Source: CAD feature listing. Evaluate the final solid. Frame: model axes, mm. Face numbers are marked on the shaded views. A direction names the side the tool comes from. Give positions to 0.01 mm unless a question says otherwise; leave off trailing zeros. Write each loop counter-clockwise with the first axis right and the second up, starting at its lowest first coordinate (ties: lowest second). Pieces come first, ordered by that corner, then holes. Notation, with made-up numbers: (81.5, -34) -> (94.5, -34) arc R32 cw to (94.5, -7) -> close; hole circle Ø9 at (76.25, 28). An arc over 180 degrees is marked (long way). Use a Markdown table: item, result. Add a question column.
```python
from build123d import *

# Parameters (mm, degrees)
SKETCH_1_W           = 80
SKETCH_1_H           = 150
EXTRUDE_1_DEPTH      = 10
SKETCH_4_R           = 11.25
EXTRUDE_3_DEPTH      = 10
SKETCH_5_R           = 11.25
SKETCH_5_R_2         = 5
EXTRUDE_4_DEPTH      = 4
SKETCH_6_R           = 2.1
CUT_EXTRUDE_1_DEPTH  = 24
SKETCH_7_W           = 3.4
SKETCH_7_H           = 7.5
CUT_EXTRUDE_2_DEPTH  = 24
SKETCH_8_R           = 2.1
CUT_EXTRUDE_3_DEPTH  = 24
SKETCH_9_W           = 80
SKETCH_9_H           = 40
SKETCH_9_R           = 11
SKETCH_9_R_2         = 1.6
EXTRUDE_5_DEPTH      = 10
FILLET_1_R           = 5
SKETCH_10_W          = 3.4
SKETCH_10_H          = 7.5
CUT_EXTRUDE_5_DEPTH  = 10
SKETCH_11_R          = 2.1
CUT_EXTRUDE_6_DEPTH  = 24
SKETCH_12_R          = 2.1
CUT_EXTRUDE_7_DEPTH  = 24
SKETCH_14_W          = 4
SKETCH_14_H          = 2
CUT_EXTRUDE_9_DEPTH  = 10
SKETCH_16_R          = 2.1
CUT_EXTRUDE_10_DEPTH = 11
CUT_EXTRUDE_12_DEPTH = 81
CUT_EXTRUDE_13_DEPTH = 3
SKETCH_20_R          = 1.6
CUT_EXTRUDE_15_DEPTH = 20


with BuildPart() as part:
    # 草圖1 → 填料-伸長1 (new body)
    with BuildSketch(Plane.XY):
        Rectangle(SKETCH_1_W, SKETCH_1_H)
    extrude(amount=EXTRUDE_1_DEPTH)

    # 草圖4 → 填料-伸長3 (add)
    with BuildSketch(Plane.XZ.offset(75)):
        with BuildLine():
            ThreePointArc((-6, 49), (0, 43), (6, 49))
            Line((6, 49), (6, 50))
            Line((6, 50), (29, 50))
            Line((29, 50), (29, 27.881405907))
            ThreePointArc((29, 27.881405907), (30, 21.95), (31, 27.881405907))
            Line((31, 27.881405907), (31, 50))
            Line((31, 50), (40, 50))
            Line((40, 50), (40, 10))
            Line((40, 10), (-40, 10))
            Line((-40, 10), (-40, 50))
            Line((-40, 50), (-31, 50))
            Line((-31, 50), (-31, 27.881405907))
            ThreePointArc((-31, 27.881405907), (-30, 21.95), (-29, 27.881405907))
            Line((-29, 27.881405907), (-29, 50))
            Line((-29, 50), (-6, 50))
            Line((-6, 50), (-6, 49))
        make_face()
        with Locations((0, 25)):
            Circle(SKETCH_4_R, mode=Mode.SUBTRACT)
    extrude(amount=-EXTRUDE_3_DEPTH)

    # 草圖5 → 填料-伸長4 (add)
    with BuildSketch(Plane.XZ.offset(75)):
        with Locations((0, 25)):
            Circle(SKETCH_5_R)
        with Locations((0, 25)):
            Circle(SKETCH_5_R_2, mode=Mode.SUBTRACT)
    extrude(amount=-EXTRUDE_4_DEPTH)

    # 草圖6 → 除料-伸長1 (cut)
    with BuildSketch(Plane(origin=(40, 0, 0), x_dir=(0, 0, -1), z_dir=(1, 0, 0))):
        with Locations((-40, -70)):
            Circle(SKETCH_6_R)
    extrude(amount=-CUT_EXTRUDE_1_DEPTH, mode=Mode.SUBTRACT)

    # 草圖7 → 除料-伸長2 (cut)
    with BuildSketch(Plane.XZ.offset(75)):
        with Locations((-21.943112787, 40)):
            Rectangle(SKETCH_7_W, SKETCH_7_H)
        with Locations((21.943112787, 40)):
            Rectangle(SKETCH_7_W, SKETCH_7_H)
    extrude(amount=-CUT_EXTRUDE_2_DEPTH, mode=Mode.SUBTRACT)

    # 草圖8 → 除料-伸長3 (cut)
    with BuildSketch(Plane.ZY.offset(40)):
        with Locations((40, -70)):
            Circle(SKETCH_8_R)
    extrude(amount=-CUT_EXTRUDE_3_DEPTH, mode=Mode.SUBTRACT)

    # 草圖9 → 填料-伸長5 (add)
    with BuildSketch(Plane(origin=(0, 75, 0), x_dir=(1, 0, 0), z_dir=(0, 1, 0))):
        with Locations((0, -30)):
            Rectangle(SKETCH_9_W, SKETCH_9_H)
        with Locations((0, -25)):
            Circle(SKETCH_9_R, mode=Mode.SUBTRACT)
        with Locations((-21.920310217, -25)):
            Circle(SKETCH_9_R_2, mode=Mode.SUBTRACT)
        with Locations((0, -46.920310217)):
            Circle(SKETCH_9_R_2, mode=Mode.SUBTRACT)
        with Locations((21.920310217, -25)):
            Circle(SKETCH_9_R_2, mode=Mode.SUBTRACT)
    extrude(amount=-EXTRUDE_5_DEPTH)

    # 圓角1
    fillet_1_edges = [part.edges().sort_by_distance(p)[0] for p in [
        (40, 70, 50),
        (-40, 70, 50),
        (40, -70, 50),
        (-40, -70, 50),
    ]]
    fillet(fillet_1_edges, radius=FILLET_1_R)

    # 草圖10 → 除料-伸長5 (cut)
    with BuildSketch(Plane(origin=(0, 75, 0), x_dir=(1, 0, 0), z_dir=(0, 1, 0))):
        with BuildLine():
            Line((-30.992105359, -72.117230176), (-29, -72.117230176))
            Line((-29, -72.117230176), (-29, -27.881405907))
            ThreePointArc((-29, -27.881405907), (-30.004176302, -21.950002859), (-30.992105359, -27.884133658))
            Line((-30.992105359, -27.884133658), (-30.992105359, -72.117230176))
        make_face()
        with BuildLine():
            Line((29.001577897, -72.118320527), (31, -72.118320527))
            Line((31, -72.118320527), (31, -27.881405907))
            ThreePointArc((31, -27.881405907), (29.999164969, -21.950000114), (29.001577897, -27.881953036))
            Line((29.001577897, -27.881953036), (29.001577897, -72.118320527))
        make_face()
        with Locations((-21.943112787, -40)):
            Rectangle(SKETCH_10_W, SKETCH_10_H)
        with Locations((21.943112787, -40)):
            Rectangle(SKETCH_10_W, SKETCH_10_H)
    extrude(amount=-CUT_EXTRUDE_5_DEPTH, mode=Mode.SUBTRACT)

    # 草圖11 → 除料-伸長6 (cut)
    with BuildSketch(Plane(origin=(40, 0, 0), x_dir=(0, 0, -1), z_dir=(1, 0, 0))):
        with Locations((-40, 70)):
            Circle(SKETCH_11_R)
    extrude(amount=-CUT_EXTRUDE_6_DEPTH, mode=Mode.SUBTRACT)

    # 草圖12 → 除料-伸長7 (cut)
    with BuildSketch(Plane.ZY.offset(40)):
        with Locations((40, 70)):
            Circle(SKETCH_12_R)
    extrude(amount=-CUT_EXTRUDE_7_DEPTH, mode=Mode.SUBTRACT)

    # 草圖14 → 除料-伸長9 (cut)
    with BuildSketch(Plane.XZ.offset(75)):
        with Locations((-12, 46)):
            Rectangle(SKETCH_14_W, SKETCH_14_H)
        with Locations((12, 46)):
            Rectangle(SKETCH_14_W, SKETCH_14_H)
    extrude(amount=-CUT_EXTRUDE_9_DEPTH, mode=Mode.SUBTRACT)

    # 草圖16 → 除料-伸長10 (cut, through all)
    with BuildSketch(Plane.XY.offset(10)):
        with Locations((-20, 37.5)):
            Circle(SKETCH_16_R)
        with Locations((20, 37.5)):
            Circle(SKETCH_16_R)
        with Locations((20, -37.5)):
            Circle(SKETCH_16_R)
        with Locations((-20, -37.5)):
            Circle(SKETCH_16_R)
    extrude(amount=-CUT_EXTRUDE_10_DEPTH, mode=Mode.SUBTRACT)

    # 草圖17 → 除料-伸長12 (cut, through all)
    with BuildSketch(Plane(origin=(40, 0, 0), x_dir=(0, 0, -1), z_dir=(1, 0, 0))):
        Polygon((-10, -15), (-13, -15), (-13, 0), (-5, 0), (-5, -15), (0, -15), (0, -75), (-50, -75), (-50, -65), (-10, -65), align=None)
    extrude(amount=-CUT_EXTRUDE_12_DEPTH, mode=Mode.SUBTRACT)

    # 草圖19 → 除料-伸長13 (cut)
    with BuildSketch(Plane(origin=(0, 0, 0), x_dir=(-1, 0, 0), z_dir=(0, 0, -1))):
        Polygon((-18.036462654, -7.5), (-19.768513462, -4.5), (-23.232615077, -4.5), (-24.964665884, -7.5), (-23.232615077, -10.5), (-19.768513462, -10.5), align=None)
        Polygon((23.464101615, -7.5), (21.732050808, -4.5), (18.267949192, -4.5), (16.535898385, -7.5), (18.267949192, -10.5), (21.732050808, -10.5), align=None)
    extrude(amount=-CUT_EXTRUDE_13_DEPTH, mode=Mode.SUBTRACT)

    # 草圖20 → 除料-伸長15 (cut)
    with BuildSketch(Plane(origin=(0, 0, 0), x_dir=(-1, 0, 0), z_dir=(0, 0, -1))):
        with Locations((-21.500564269, -7.5)):
            Circle(SKETCH_20_R)
        with Locations((20, -7.5)):
            Circle(SKETCH_20_R)
    extrude(amount=-CUT_EXTRUDE_15_DEPTH, mode=Mode.SUBTRACT)


solid = part.part
```
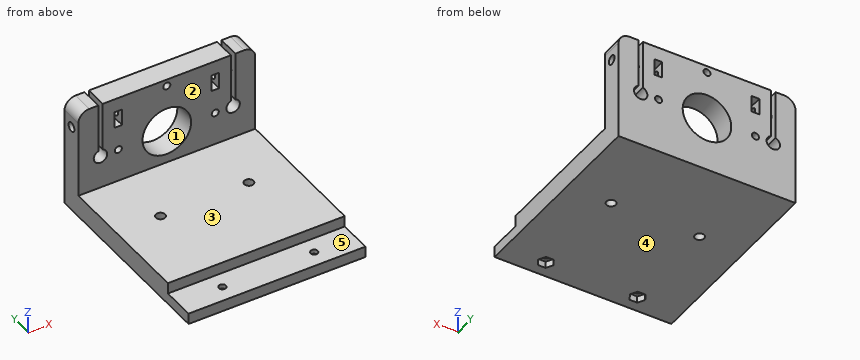
(1) Mould query, pull axis Z, two halves, no side actions, for the marked faces 1, 2 and 3. Classes: +Z half, -Z half, draft (parallel to the pull), parting line (faces both ways), or undercut.
(2) Cut plane A-A on x = 0. Return the cut outline in (y, z).
(3) Material intervals for L1, parallel to X at y = 69.5, z = 25; L2, parallel to Y at x = -20, z = 4.35; L3, parallel to Y at x = -27.3, z = 40, sorted ascending.
(4) Cut plane C-C on z = 20. Return the cut outline in (x, y).
(5) Cut plane D-D on z = 29. Return the cut outline in (x, y).
(6) First-contact query: pin 1 Ø12 at (y, z) = (20.5, 18.5) entering from -X; pin 2 Ø3 at (x, y) = (19, 63) entering from +Z; pin 3 Ø4 at (x, z) = (-11.5, 12.5) entering from -Y; pin 4 Ø2 at (y, z) = (69.5, 39.5) entering from +X. Flat tips, straight axial feed; report the tip coordinate or a pass-through.
(7) Cut plane B-B on y = 37.5. Return the cut outline in (x, z).
(8) Access query for the marked faces 4 and 5. Directions: +Z, -Z, +X, -X, +Y, -Y. A direction counts if a zero-diameter tool reaches every point of the face in a straight line with its end or side. Return the directions, or none.
Output:
| question | item | result |
|---|---|---|
| 1 | face 1 | undercut |
| 1 | face 2 | draft |
| 1 | face 3 | +Z half |
| 2 | outline | (-15, 0) -> (75, 0) -> (75, 14) -> (65, 14) -> (65, 10) -> (0, 10) -> (0, 5) -> (-15, 5) -> close; (65, 36) -> (75, 36) -> (75, 45.32) -> (65, 45.32) -> close; (65, 48.52) -> (75, 48.52) -> (75, 50) -> (65, 50) -> close |
| 3 | L1 | -40 to -33.05, -26.95 to -23.52, -20.32 to -11, 11 to 20.32, 23.52 to 26.95, 33.05 to 40 |
| 3 | L2 | -15 to -9.1, -5.9 to 35.4, 39.6 to 75 |
| 3 | L3 | 65 to 67.9, 72.1 to 75 |
| 4 | outline | (-40, 65) -> (-9.8, 65) -> (-9.8, 75) -> (-40, 75) -> close; (9.8, 65) -> (40, 65) -> (40, 75) -> (9.8, 75) -> close |
| 5 | outline | (-40, 65) -> (-30.99, 65) -> (-30.99, 75) -> (-40, 75) -> close; (-29, 65) -> (-10.25, 65) -> (-10.25, 75) -> (-29, 75) -> close; (10.25, 65) -> (29, 65) -> (29, 75) -> (10.25, 75) -> close; (31, 65) -> (40, 65) -> (40, 75) -> (31, 75) -> close |
| 6 | pin 1 | through |
| 6 | pin 2 | z = 10 |
| 6 | pin 3 | y = 65 |
| 6 | pin 4 | x = 16 |
| 7 | outline | (-40, 0) -> (-22.1, 0) -> (-22.1, 10) -> (-40, 10) -> close; (-17.9, 0) -> (17.9, 0) -> (17.9, 10) -> (-17.9, 10) -> close; (22.1, 0) -> (40, 0) -> (40, 10) -> (22.1, 10) -> close |
| 8 | face 4 | -Z, +X, -X, +Y, -Y |
| 8 | face 5 | +Z, +X, -X, -Y |
